Check sheet for the modelled part. Datum: model origin and axes. Units: mm. Face numbers are marked on the shaded views. A direction names the side the tool comes from. Give positions to 0.01 mm unless a question says otherwise; leave off trailing zeros. Order: outer loops, then holes, each group sorted by start corner. A loop starts at its lowest first (then second) coordinate and runs counter-clockwise, first axis right, second up. Notation, with made-up numbers: (87.5, 28.5) -> (135.5, 28.5) arc R11 cw to (135.5, 32.5) -> close; hole circle Ø4 at (-23, 38.5). An arc over 180 degrees is marked (long way). Answer in a Markdown table with one row per item. Add a question column.
(1) Cross-section at C-C (z = 162.5). Record the cut outline in (x, y), then the cut area to 3 significant figures.
(2) Set-up check for the marked faces 1 and 2: record each of +Z, -Z, +X, -X, +Y, -Y from which the full face is reachable in a straight line by a thin tool's end or side.
(3) Cross-section at D-D (z = 62.5). Record the cut outline in (x, y), then the cut area to 3 significant figures.
(4) Cross-section at A-A (x = 0). Record the cut outline in (y, z).
(5) Thickness scan on L1, parallel to Y at x = 6.75, z = 168; L2, parallel to X at y = 8, z = 175; L3, parallel to Y at x = -0.5, z = 102.5. Record the ranges inside material, lowest first. Write a range as [from, to].
(6) Go/stop test with flat-tipped pins: pin 1 (1.5 mm diameter, centred on y = 5, z = 129, fed in from +X); pin 2 (4 mm diameter, centred on x = 2.5, z = 86, fed in from +Y); pin 3 (8 mm diameter, centred on x = 5, y = 0.5, fed in from +Z); pin 4 (7 mm diameter, centred on x = 0, z = 175, fed in from -Y). Record where each tip stops, or that it passes through.
(7) Cross-section at B-B (y = -8). Record the cut outline in (x, z).
```python
from build123d import *

# Parameters (mm, degrees)
SKETCH_2_R          = 10
EXTRUDE_1_DEPTH     = 150
SKETCH_3_W          = 20
SKETCH_3_H          = 25
EXTRUDE_2_DEPTH     = 35
SKETCH_4_W          = 60
SKETCH_4_H          = 10
CUT_EXTRUDE_1_DEPTH = 50
SKETCH_5_R          = 4
CUT_EXTRUDE_2_DEPTH = 50
FILLET_3_RADIUS     = 10
FILLET_3_LENGTH     = 7.5
FILLET_4_RADIUS     = 10
FILLET_4_LENGTH     = 7.5


with BuildPart() as part:
    # 草图2 → 凸台-拉伸1 (new body)
    with BuildSketch(Plane.XY):
        Circle(SKETCH_2_R)
    extrude(amount=EXTRUDE_1_DEPTH)

    # 草图3 → 凸台-拉伸2 (add)
    with BuildSketch(Plane.XY.offset(150)):
        Rectangle(SKETCH_3_W, SKETCH_3_H)
    extrude(amount=EXTRUDE_2_DEPTH)

    # 草图4 → 切除-拉伸1 (cut)
    with BuildSketch(Plane.ZY.offset(10)):
        with Locations((185, 0)):
            Rectangle(SKETCH_4_W, SKETCH_4_H)
    extrude(amount=-CUT_EXTRUDE_1_DEPTH, mode=Mode.SUBTRACT)

    # 草图5 → 切除-拉伸2 (cut)
    with BuildSketch(Plane.XZ.offset(12.5)):
        with Locations(Location((0, 175, 0), (0, 0, 270))):
            Circle(SKETCH_5_R)
    extrude(amount=-CUT_EXTRUDE_2_DEPTH, mode=Mode.SUBTRACT)

    # 圆角3: full round fillet: the end face becomes a half cylinder, R = half its width
    fillet_3_face = Plane((0, -8.75, 185), x_dir=(0, -1, 0), z_dir=(0, 0, 1))  # on the end face: x along it, z out of the body
    fillet_3_slab = fillet_3_face.offset(-FILLET_3_RADIUS / 2) * Box(FILLET_3_LENGTH, 2 * FILLET_3_RADIUS, FILLET_3_RADIUS, mode=Mode.PRIVATE)  # the body's end, R deep
    fillet_3_round = Plane((0, -8.75, 175), x_dir=(0, 0, 1), z_dir=(0, -1, 0)) * Cylinder(FILLET_3_RADIUS, FILLET_3_LENGTH, mode=Mode.PRIVATE)  # its axis R under the face
    add(fillet_3_slab - fillet_3_round, mode=Mode.SUBTRACT)

    # 圆角4: full round fillet: the end face becomes a half cylinder, R = half its width
    fillet_4_face = Plane((0, 8.75, 185), x_dir=(0, 1, 0), z_dir=(0, 0, 1))  # on the end face: x along it, z out of the body
    fillet_4_slab = fillet_4_face.offset(-FILLET_4_RADIUS / 2) * Box(FILLET_4_LENGTH, 2 * FILLET_4_RADIUS, FILLET_4_RADIUS, mode=Mode.PRIVATE)  # the body's end, R deep
    fillet_4_round = Plane((0, 8.75, 175), x_dir=(0, 0, 1), z_dir=(0, 1, 0)) * Cylinder(FILLET_4_RADIUS, FILLET_4_LENGTH, mode=Mode.PRIVATE)  # its axis R under the face
    add(fillet_4_slab - fillet_4_round, mode=Mode.SUBTRACT)


solid = part.part
```
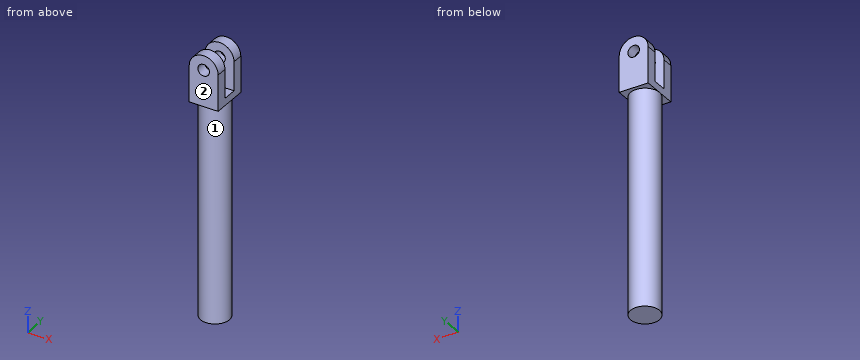
Answer below:
| question | item | result |
|---|---|---|
| 1 | outline | (-10, -12.5) -> (10, -12.5) -> (10, -5) -> (-10, -5) -> close; (-10, 5) -> (10, 5) -> (10, 12.5) -> (-10, 12.5) -> close |
| 1 | area | 300 mm² |
| 2 | face 1 | -Z |
| 2 | face 2 | +Z, -Z, +X, -X, -Y |
| 3 | outline | circle Ø20 at (0, 0) |
| 3 | area | 314 mm² |
| 4 | outline | (-12.5, 150) -> (-10, 150) -> (-10, 0) -> (10, 0) -> (10, 150) -> (12.5, 150) -> (12.5, 171) -> (5, 171) -> (5, 155) -> (-5, 155) -> (-5, 171) -> (-12.5, 171) -> close; (-12.5, 179) -> (-5, 179) -> (-5, 185) -> (-12.5, 185) -> close; (5, 179) -> (12.5, 179) -> (12.5, 185) -> (5, 185) -> close |
| 5 | L1 | y = [-12.5, -5], [5, 12.5] |
| 5 | L2 | x = [-10, -4], [4, 10] |
| 5 | L3 | y = [-9.99, 9.99] |
| 6 | pin 1 | stops at x = 9.05 |
| 6 | pin 2 | stops at y = 9.99 |
| 6 | pin 3 | stops at z = 155 |
| 6 | pin 4 | passes through |
| 7 | outline | (-10, 150) -> (-6, 150) -> (-6, 0) -> (6, 0) -> (6, 150) -> (10, 150) -> (10, 175) arc R10 ccw to (-10, 175) -> close; hole circle Ø8 at (0, 175) |
